Could you check a few things on this model? Use its own coordinates, in mm. A direction names the side the tool comes from. Coordinates: 2 decimals unless noted, no trailing zeros. Loops run counter-clockwise (first coordinate to the right, second up) from the corner with the lowest first, then second, coordinate; pieces in that order, holes last. Notation, with made-up numbers: M 23.25,77 L 27.25,77 A20 cw 27.25,107 Z; hole C -28.5,66 d1. An arc over 180 degrees is marked long. Write each question's results on one line, items separated by ' | '.
```python
from build123d import *

# Parameters (mm, degrees)
F0_R     = 1.5
F0_R_2   = 3.5
F0_W     = 10
F0_H     = 7
F0_R_3   = 2.5
F1_DEPTH = 3.175


with BuildPart() as f1:
    # F0 (on Top) → F1 (new body)
    with BuildSketch(Plane.XY):
        with BuildLine():
            Line((-170.709795, 149.497605), (-160.021436, 138.6452))
            Line((-160.021436, 138.6452), (-160.021436, 15.045131))
            ThreePointArc((-160.021436, 15.045131), (-175.04201, -0.012286), (-159.996863, -15.045151))
            Line((-159.996863, -15.045151), (-159.996863, -138.64522))
            Line((-159.996863, -138.64522), (-170.709795, -149.497605))
            ThreePointArc((-170.709795, -149.497605), (-170.62604, -170.587128), (-149.536967, -170.748253))
            Line((-149.536967, -170.748253), (-138.843533, -159.876655))
            Line((-138.843533, -159.876655), (-15.243465, -159.876655))
            ThreePointArc((-15.243465, -159.876655), (0.163697, -175.119241), (15.239949, -159.549279))
            Line((15.239949, -159.549279), (138.840017, -159.549279))
            Line((138.840017, -159.549279), (149.536967, -170.748253))
            ThreePointArc((149.536967, -170.748253), (170.62604, -170.587128), (170.709795, -149.497605))
            Line((170.709795, -149.497605), (160.003137, -138.307913))
            Line((160.003137, -138.307913), (160.003137, -14.707844))
            ThreePointArc((160.003137, -14.707844), (174.71038, -0.133012), (160.269149, 14.705439))
            Line((160.269149, 14.705439), (160.269149, 138.305507))
            Line((160.269149, 138.305507), (170.709795, 149.497605))
            ThreePointArc((170.709795, 149.497605), (170.62604, 170.587128), (149.536967, 170.748253))
            Line((149.536967, 170.748253), (138.622064, 160.018153))
            Line((138.622064, 160.018153), (15.021996, 160.018153))
            ThreePointArc((15.021996, 160.018153), (0.052596, 175.145617), (-15.022364, 160.123345))
            Line((-15.022364, 160.123345), (-138.622432, 160.123345))
            Line((-138.622432, 160.123345), (-149.536967, 170.748253))
            ThreePointArc((-149.536967, 170.748253), (-170.62604, 170.587128), (-170.709795, 149.497605))
        make_face()
        with Locations((-160, -160)):
            Circle(F0_R, mode=Mode.SUBTRACT)
        with Locations((-102.589366, -102.108729)):
            Circle(F0_R, mode=Mode.SUBTRACT)
        with Locations((-76.5, -145)):
            Circle(F0_R_2, mode=Mode.SUBTRACT)
        Polygon((-15.040643, -130.069532), (-108.810426, -130.028952), (-28.798405, -50.016931), (-15.000023, -50.016931), align=None, mode=Mode.SUBTRACT)
        Polygon((-50.026811, -28.803403), (-130.038832, -108.815424), (-130.079413, -15.045641), (-50.026811, -15.005021), align=None, mode=Mode.SUBTRACT)
        with Locations((-159.996863, 0)):
            Circle(F0_R, mode=Mode.SUBTRACT)
        with Locations((-102.589366, 0)):
            Circle(F0_R, mode=Mode.SUBTRACT)
        with Locations((-10, -8)):
            Rectangle(F0_W, F0_H, mode=Mode.SUBTRACT)
        with Locations((0, -159.876655)):
            Circle(F0_R, mode=Mode.SUBTRACT)
        with Locations((76.5, -145)):
            Circle(F0_R_2, mode=Mode.SUBTRACT)
        with Locations((0, -102.108729)):
            Circle(F0_R, mode=Mode.SUBTRACT)
        Polygon((28.809005, -50.016034), (108.821026, -130.028055), (15.051243, -130.068635), (15.010623, -50.016034), align=None, mode=Mode.SUBTRACT)
        with Locations((160, -160)):
            Circle(F0_R, mode=Mode.SUBTRACT)
        with Locations((102.589366, -102.108729)):
            Circle(F0_R, mode=Mode.SUBTRACT)
        with Locations((10, -8)):
            Rectangle(F0_W, F0_H, mode=Mode.SUBTRACT)
        Circle(F0_R, mode=Mode.SUBTRACT)
        Polygon((130.052601, -15.029035), (130.012021, -108.798818), (50, -28.786797), (50, -14.988415), align=None, mode=Mode.SUBTRACT)
        with Locations((102.589366, 0)):
            Circle(F0_R, mode=Mode.SUBTRACT)
        with Locations((159.996863, 0)):
            Circle(F0_R, mode=Mode.SUBTRACT)
        Polygon((-130.021436, 14.063299), (-130.021436, 107.833091), (-49.968824, 27.861681), (-49.968824, 14.063299), align=None, mode=Mode.SUBTRACT)
        with Locations((-10, 8)):
            Rectangle(F0_W, F0_H, mode=Mode.SUBTRACT)
        with Locations((-102.589366, 102.108729)):
            Circle(F0_R, mode=Mode.SUBTRACT)
        with Locations((-160, 160)):
            Circle(F0_R, mode=Mode.SUBTRACT)
        Polygon((-28.785476, 50.070734), (-108.756886, 130.123345), (-14.987094, 130.123345), (-14.987094, 50.070734), align=None, mode=Mode.SUBTRACT)
        with Locations((-76.5, 145.108729)):
            Circle(F0_R_3, mode=Mode.SUBTRACT)
        with Locations((10, 8)):
            Rectangle(F0_W, F0_H, mode=Mode.SUBTRACT)
        Polygon((50.521991, 28.76451), (130.493401, 108.817121), (130.574562, 15.047365), (50.521991, 14.966128), align=None, mode=Mode.SUBTRACT)
        with Locations((0, 102.108729)):
            Circle(F0_R, mode=Mode.SUBTRACT)
        Polygon((15.498815, 130.018728), (109.268607, 130.018728), (29.297197, 49.966116), (15.498815, 49.966116), align=None, mode=Mode.SUBTRACT)
        with Locations((0, 160.723508)):
            Circle(F0_R, mode=Mode.SUBTRACT)
        with Locations((76.5, 145.108729)):
            Circle(F0_R_3, mode=Mode.SUBTRACT)
        with Locations((102.589366, 102.108729)):
            Circle(F0_R, mode=Mode.SUBTRACT)
        with Locations((160, 160)):
            Circle(F0_R, mode=Mode.SUBTRACT)
    extrude(amount=F1_DEPTH)


solid = f1.part
```
(1) Please list where these lines run through material, in increasing order: probe 1 along Y at (x, z) = (0, 0.75); probe 2 along Y at (x, z) = (-88.5, 0.45); probe 3 along X at (y, z) = (127.5, 2.8). Write a range as from..to.
Reported:
probe 1: y = -175.12..-161.38, -158.38..-103.61, -100.61..-1.5, 1.5..100.61, 103.61..159.22, 162.22..175.15 | probe 2: y = -159.88..-130.04, -109.72..-67.28, -15.02..14.06, 66.35..109.85, 130.12..160.12 | probe 3: x = -160.02..-106.14, -14.99..15.5, 106.75..160.27
(2) Imagine slicing it at C-C, the plane z = 2.65. State how many separate pieces and enclosed holes the cut face has, and give its area (3 significant figures).
Reported:
separate pieces: 1 | enclosed holes: 33 | area: 71,200 mm2
(3) Which directions (+Z, -Z, +X, -X, +Y, -Y) give clear straight access to the entire face, cutting with the end or side of a thin tool? Please do faces 4 (the flat face through (-144.265, -165.389, 1.565)), 5 (the flat face through (-89.473, -68.249, 1.565)), 6 (the flat face through (-165.278, -143.995, 1.565)).
Reported:
face 4: +Z, -Z, -Y | face 5: +Z, -Z | face 6: +Z, -Z, -X
(4) If we mould it in two halves opening along Y, with no side actions, what happens to faces 1 (the flat face through (-2, 2, 3.175)), 2 (the flat face through (68.255, -89.462, 1.565)), 3 (the flat face through (144.2, 165.5, 1.6))? For each: released by +Y, released by -Y, zero draft, split by the parting line, or undercut.
Reported:
face 1: zero draft | face 2: undercut | face 3: released by +Y
(5) Imagine slicing it at B-B, the plane x = -34. List the corners of the cut face in (y, z) for me (3 decimals).
Reported:
outline: M -159.877,0 L -130.061,0 L -130.061,3.175 L -159.877,3.175 Z; M -55.219,0 L 55.291,0 L 55.291,3.175 L -55.219,3.175 Z; M 130.123,0 L 160.123,0 L 160.123,3.175 L 130.123,3.175 Z
(6) Imagine slicing it at A-A, the plane y = 92. List the corners of the cut face in (x, z) for me (3 decimals), and give its area (3 significant figures).
Reported:
outline: M -160.021,0 L -130.021,0 L -130.021,3.175 L -160.021,3.175 Z; M -114.172,0 L -70.672,0 L -70.672,3.175 L -114.172,3.175 Z; M -14.987,0 L 15.499,0 L 15.499,3.175 L -14.987,3.175 Z; M 71.288,0 L 113.693,0 L 113.693,3.175 L 71.288,3.175 Z; M 130.508,0 L 160.269,0 L 160.269,3.175 L 130.508,3.175 Z | area: 559 mm2
(7) Will these pins go through, and if not, where does the flat tip stop? P1, Ø1, axis at x = 9.5, z = 1, coming from the +Y side; P2, Ø1.5, axis at y = -23, z = 1, coming from the -X side; P3, Ø1, axis at x = -65.5, z = 1.5, coming from the -Y side.
Reported:
P1: stops at y = 172.15 | P2: stops at x = -160 | P3: stops at y = -159.88
